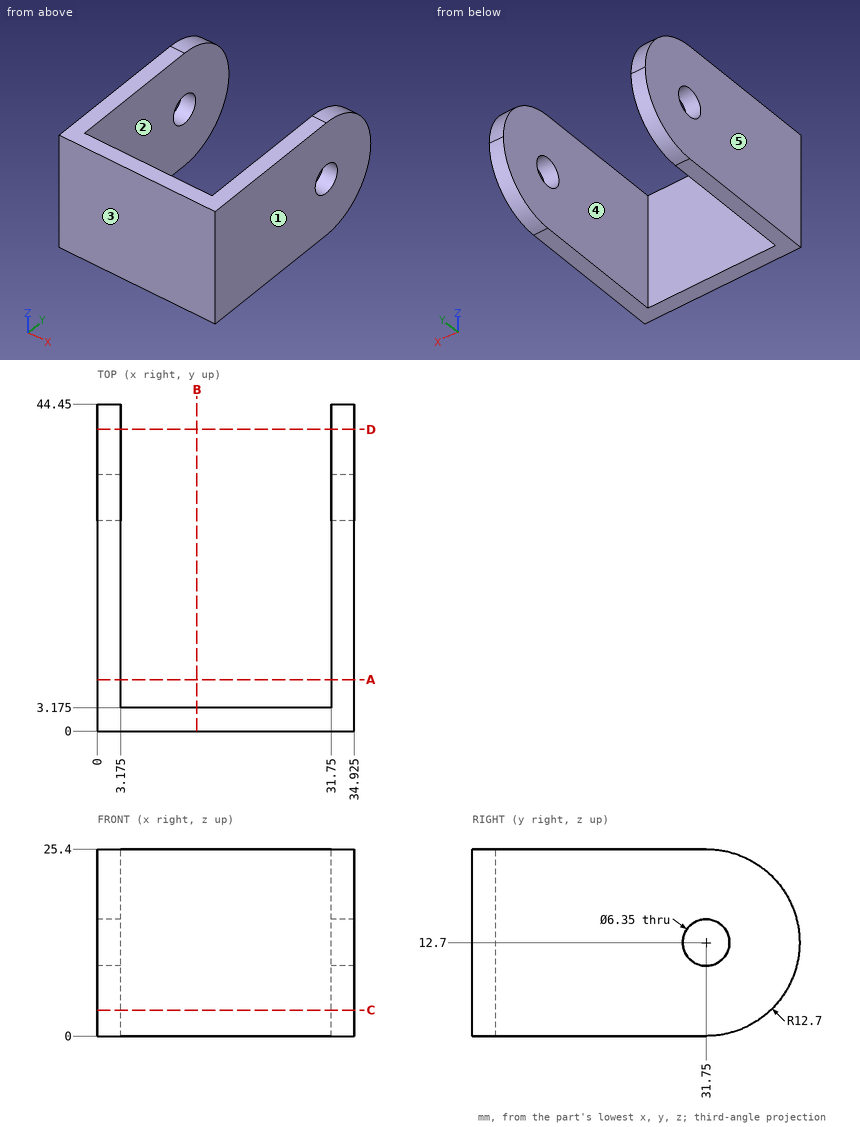
Geometry: see drawing. Coordinates: mm, zero at the bounding-box minimum. A direction names the side the tool comes from. Round coordinates to 2 decimals unless told otherwise and drop trailing zeros. Loops run counter-clockwise (first coordinate to the right, second up) from the corner with the lowest first, then second, coordinate; pieces in that order, holes last. Notation, with made-up numbers: (3.25, -13.5) -> (9.25, -13.5) arc R32 cw to (9.25, 12.5) -> close; hole circle Ø3 at (-33.75, 55.25). An arc over 180 degrees is marked (long way). Write each question's results on one line, items separated by ' | '.
1. Section B-B (x = 13.5). Return loops of the section in (y, z) (3 decimals).
Geometry results:
outline: (0, 0) -> (3.175, 0) -> (3.175, 25.4) -> (0, 25.4) -> close
2. Set-up query: the marked faces 4 and 5. Return all of +Z, -Z, +X, -X, +Y, -Y with unobstructed straight access to the full face (end or side cutting, diameter ignored); none if empty.
Geometry results:
face 4: +Z, -Z, +Y | face 5: +Z, -Z, -X, +Y, -Y
3. Section D-D (y = 41). Return loops of the section in (x, z) (3 decimals).
Geometry results:
outline: (0, 3.998) -> (3.175, 3.998) -> (3.175, 21.402) -> (0, 21.402) -> close; (31.75, 3.998) -> (34.925, 3.998) -> (34.925, 21.402) -> (31.75, 21.402) -> close
4. Section C-C (z = 3.5). Return loops of the section in (x, y) (3 decimals).
Geometry results:
outline: (0, 0) -> (34.925, 0) -> (34.925, 40.505) -> (31.75, 40.505) -> (31.75, 3.175) -> (3.175, 3.175) -> (3.175, 40.505) -> (0, 40.505) -> close
5. First-contact query: P1, Ø4, axis at x = 5, z = 9.5, coming from the +Y side. Flat tip, straight axial feed; report the tip coordinate or a pass-through.
Geometry results:
P1: y = 44.22
6. Ray query, line 1 (X direction, y = 5, z = 17.25) (3 decimals); line 2 (Y direction, x = 19.5, z = 14.25) (3 decimals); line 3 (Z direction, x = 33, y = 31). Return the intervals inside material, ascending. Write a range as from..to.
Geometry results:
line 1: 0..3.175, 31.75..34.925 | line 2: 0..3.175 | line 3: 0..9.61, 15.79..25.4
7. Mould query, pull axis X, two halves, no side actions, for the marked faces 1, 2 and 3. Classes: +X half, -X half, draft (parallel to the pull), parting line (faces both ways), or undercut.
Geometry results:
face 1: +X half | face 2: undercut | face 3: draft
8. Section A-A (y = 7). Return loops of the section in (x, z) (3 decimals), and give its area (3 significant figures).
Geometry results:
outline: (0, 0) -> (3.175, 0) -> (3.175, 25.4) -> (0, 25.4) -> close; (31.75, 0) -> (34.925, 0) -> (34.925, 25.4) -> (31.75, 25.4) -> close | area: 161 mm2
